Can you work these out from the model? Positions are in its coordinate system, mm. Round coordinates to 2 decimals unless told otherwise and drop trailing zeros. Write each loop counter-clockwise with the first axis right and the second up, starting at its lowest first coordinate (ties: lowest second). Pieces come first, ordered by that corner, then holes. Notation, with made-up numbers: (21, -30.75) -> (67, -30.75) arc R15 cw to (67, -8.75) -> close; hole circle Ø9 at (-31, 53). An arc over 180 degrees is marked (long way). Write item = value, one per line. Start each with the question number.
1) If I drill on line 1 (X direction, y = 2.8, z = 0); line 2 (Z direction, x = -33.5, y = 1.95); line 3 (Z direction, x = -9.5, y = 2.1), over which ranges is the centre line in solid material (lowest first)?
2) Imagine slicing it at D-D, the plane x = -11. Please give me the cut outline in (y, z).
3) Imagine slicing it at B-B, the plane z = 0. Please give me the cut outline in (x, y).
4) Imagine slicing it at A-A, the plane x = 32.5. Please give me the cut outline in (y, z), then the cut area to 3 significant figures.
5) Imagine slicing it at C-C, the plane y = 2.4. Please give me the cut outline in (x, z), then the cut area to 3 significant figures.
from build123d import *

# Parameters (mm, degrees)
SKETCH1_W           = 80.830931362
SKETCH1_H           = 33.48304161
SKETCH1_R           = 2.032
BOSS_EXTRUDE1_DEPTH = 3.302
SKETCH2_R           = 3.96875
SKETCH2_R_2         = 2.286
CUT_EXTRUDE1_DEPTH  = 3.302


with BuildPart() as part:
    # Sketch1 → Boss-Extrude1 (new body)
    with BuildSketch(Plane(origin=(0, 0, 0), x_dir=(1, 0, 0), z_dir=(0, 1, 0))):
        Rectangle(SKETCH1_W, SKETCH1_H)
        with Locations(Location((-33.401, 0, 0), (0, 0, 90))):
            Circle(SKETCH1_R, mode=Mode.SUBTRACT)
        with Locations(Location((33.401, 0, 0), (0, 0, 90))):
            Circle(SKETCH1_R, mode=Mode.SUBTRACT)
    extrude(amount=BOSS_EXTRUDE1_DEPTH)

    # Sketch2 → Cut-Extrude1 (cut)
    with BuildSketch(Plane.XZ):
        with Locations(Location((-9.4615, 0, 0), (0, 0, 270))):
            Circle(SKETCH2_R)
        with Locations(Location((22.209125, 0.016190079, 0), (0, 0, 270))):
            Circle(SKETCH2_R_2)
    extrude(amount=-CUT_EXTRUDE1_DEPTH, mode=Mode.SUBTRACT)


solid = part.part
Reported:
q1.line_1 = -40.42 to -35.43, -31.37 to -13.43, -5.49 to 19.92, 24.5 to 31.37, 35.43 to 40.42
q1.line_2 = -16.74 to -2.03, 2.03 to 16.74
q1.line_3 = -16.74 to -3.97, 3.97 to 16.74
q2.outline = (0, -16.74) -> (3.3, -16.74) -> (3.3, -3.66) -> (0, -3.66) -> close; (0, 3.66) -> (3.3, 3.66) -> (3.3, 16.74) -> (0, 16.74) -> close
q3.outline = (-40.42, 0) -> (-35.43, 0) -> (-35.43, 3.3) -> (-40.42, 3.3) -> close; (-31.37, 0) -> (-13.43, 0) -> (-13.43, 3.3) -> (-31.37, 3.3) -> close; (-5.49, 0) -> (19.92, 0) -> (19.92, 3.3) -> (-5.49, 3.3) -> close; (24.5, 0) -> (31.37, 0) -> (31.37, 3.3) -> (24.5, 3.3) -> close; (35.43, 0) -> (40.42, 0) -> (40.42, 3.3) -> (35.43, 3.3) -> close
q4.outline = (0, -16.74) -> (3.3, -16.74) -> (3.3, -1.82) -> (0, -1.82) -> close; (0, 1.82) -> (3.3, 1.82) -> (3.3, 16.74) -> (0, 16.74) -> close
q4.area = 98.5 mm²
q5.outline = (-40.42, -16.74) -> (40.42, -16.74) -> (40.42, 16.74) -> (-40.42, 16.74) -> close; hole circle Ø4.06 at (-33.4, 0); hole circle Ø7.94 at (-9.46, 0); hole circle Ø4.57 at (22.21, 0.02); hole circle Ø4.06 at (33.4, 0)
q5.area = 2,610 mm²
